Geometry: final body of the model. Coordinates: model frame, mm. Coordinates: 2 decimals unless noted, no trailing zeros. Write item = value, one per line. Start each with the question number.
Autodesk Inventor part; units mm, degrees
ref_plane "YZ Plane" through (0, 0, 0) normal (1, 0, 0) x (0, 1, 0)
ref_plane "XZ Plane" through (0, 0, 0) normal (0, 1, 0) x (-1, 0, 0)
ref_plane "XY Plane" through (0, 0, 0) normal (0, 0, 1) x (1, 0, 0)
sketch "Sketch1" plane through (0, 0, 0) normal (0, 0, 1) x (1, 0, 0)
  line L0 (0, -144.3376) -> (-125, 72.1688) construction
  line L1 (-125, 72.1688) -> (125, 72.1688) construction
  line L2 (125, 72.1688) -> (0, -144.3376) construction
  line L3 (0, 173.2051) -> (150, -86.6025) construction
  line L4 (150, -86.6025) -> (-150, -86.6025) construction
  line L5 (-150, -86.6025) -> (0, 173.2051) construction
  circle A0 centre (-150, -86.6025) radius 1.5875
  circle A1 centre (150, -86.6025) radius 1.5875
  circle A2 centre (0, 173.2051) radius 1.5875
  circle A3 centre (-125, 72.1688) radius 4.25
  circle A4 centre (125, 72.1688) radius 4.25
  circle A5 centre (0, -144.3376) radius 4.25
  circle A6 centre (-150, -86.6025) radius 25 construction
  line L6 (-250.0151, -144.3463) -> (0, 288.6926) construction
  line L7 (0, 288.6926) -> (250.0151, -144.3463) construction
  line L8 (250.0151, -144.3463) -> (-250.0151, -144.3463) construction
  arc A7 (-225.5835, -102.5089) -> (-201.5671, -144.1066) centre (-197.7721, -114.1838) ccw
  circle A8 centre (-125, 72.1688) radius 12.5 construction
  arc A9 (24.0164, 246.6155) -> (-24.0164, 246.6155) centre (0, 228.3676) ccw
  arc A10 (201.5671, -144.1066) -> (225.5835, -102.5089) centre (197.7721, -114.1838) ccw
  arc A11 (-24.0164, 246.6155) -> (-225.5835, -102.5089) centre (1251.5935, -722.6079) ccw
  arc A12 (225.5835, -102.5089) -> (24.0164, 246.6155) centre (-1251.5935, -722.6079) ccw
  arc A13 (-201.5671, -144.1066) -> (201.5671, -144.1066) centre (0, 1445.2157) ccw
  circle A14 centre (0, 228.3676) radius 1.5875
  circle A15 centre (-197.7721, -114.1838) radius 1.5875
  circle A16 centre (197.7721, -114.1838) radius 1.5875
  point P0 (0, 0)
  point P1 (0, 0)
  point P2 (0, 0)
  point P3 (0, 0)
  dimension "d0" = 300
  dimension "d1" = 250
  dimension "d2" = 3.175
  dimension "d3" = 8.5
  dimension "d4" = 50
  dimension "d5" = 60.325
  dimension "d6" = 25
  dimension "d9" = 3.175
extrude "Extrusion2" add sketch "Sketch1" along normal blind 12.5 contours A3 | A4 | A5 | A11 A9 A12 A10 A13 A7
sketch "Sketch8" plane through (0, 0, 12.5) normal (0, 0, 1) x (1, 0, 0)
  circle A0 centre (0, 173.2051) radius 1.5875
  line L0 (15.5, 157.7051) -> (-15.5, 157.7051) construction
  line L1 (-15.5, 157.7051) -> (-15.5, 188.7051) construction
  line L2 (-15.5, 188.7051) -> (15.5, 188.7051) construction
  line L3 (15.5, 188.7051) -> (15.5, 157.7051) construction
  circle A1 centre (-15.5, 157.7051) radius 1.6
  circle A2 centre (15.5, 188.7051) radius 1.6
  point P0 (0, 0)
  dimension "d34" = 3.2
  dimension "d36" = 31
extrude "Extrusion9" cut sketch "Sketch8" against normal through all contours A1 | A2
pattern_circular "Circular Pattern1" count 3 over 360 about axis through (0, 0, -10) along (0, 0, 1) of "Extrusion9"
sketch "Sketch9" plane through (0, 0, 0) normal (0, 0, -1) x (-1, 0, 0)
  circle A0 centre (43.0398, -61.7471) radius 1.621
  circle A1 centre (11.3411, 93.1567) radius 1.621
  circle A2 centre (-31.9602, 68.1567) radius 1.621
  circle A3 centre (86.3411, -36.7471) radius 1.621
  line L0 (-76.356, 80.0525) -> (31.144, -106.143)
  line L1 (31.144, -106.143) -> (130.7369, -48.643)
  line L2 (130.7369, -48.643) -> (23.2369, 137.5525)
  line L3 (23.2369, 137.5525) -> (-76.356, 80.0525)
  line L4 (-51.5025, -76.895) -> (-72.9929, -89.3025)
  arc A4 (-79.8231, -87.4724) -> (-72.9929, -89.3025) centre (-75.4929, -84.9724) ccw
  line L5 (-79.8231, -87.4724) -> (-115.6621, -25.3974)
  arc A5 (-113.8319, -18.5673) -> (-115.6621, -25.3974) centre (-111.3319, -22.8974) ccw
  line L6 (-113.8319, -18.5673) -> (-92.3415, -6.1598)
  arc A6 (-85.5114, -7.9899) -> (-92.3415, -6.1598) centre (-89.8415, -10.4899) ccw
  line L7 (-85.5114, -7.9899) -> (-49.6724, -70.0649)
  arc A7 (-51.5025, -76.895) -> (-49.6724, -70.0649) centre (-54.0025, -72.5649) ccw
  circle A8 centre (-41.0253, -76.0422) radius 1.5
  circle A9 centre (-78.9702, -97.9497) radius 1.5
  circle A10 centre (-86.3643, 2.4873) radius 1.5
  arc A11 (-125.8092, -16.8221) -> (-126.9072, -20.9202) centre (-124.3092, -19.4202) ccw
  line L8 (-126.9072, -20.9202) -> (-81.5682, -99.4497)
  arc A12 (-81.5682, -99.4497) -> (-77.4702, -100.5477) centre (-78.9702, -97.9497) ccw
  line L9 (-77.4702, -100.5477) -> (-39.5253, -78.6402)
  arc A13 (-39.5253, -78.6402) -> (-38.4272, -74.5422) centre (-41.0253, -76.0422) ccw
  line L10 (-38.4272, -74.5422) -> (-83.7662, 3.9873)
  arc A14 (-83.7662, 3.9873) -> (-87.8643, 5.0854) centre (-86.3643, 2.4873) ccw
  line L11 (-87.8643, 5.0854) -> (-125.8092, -16.8221)
  circle A15 centre (-124.3092, -19.4202) radius 1.5
  point P0 (0, 0)
extrude "Extrusion10" cut sketch "Sketch9" against normal through all contours A0 | A1 | A2 | A3 | A8 | A9 | A10 | A15
fillet "Fillet2" radius 6.35 6 edges at (0, 258.5301, 0) (135.8253, 78.4188, 0) (223.8936, -129.265, 0) (0, -156.8376, 0) (-223.8936, -129.265, 0) (-135.8253, 78.4188, 0)
sketch "Sketch2" plane through (0, 0, 12.5) normal (0, 0, 1) x (1, 0, 0)
  circle A0 centre (0, 0) radius 105
  dimension "d12" = 210
sketch "Sketch3" plane through (0, 0, 10.595) normal (0, 0, 1) x (1, 0, 0)
  circle A0 centre (0, 0) radius 105
  line L0 (-31.25, 100.2419) -> (-31.25, 30)
  line L1 (-31.25, 30) -> (31.25, 30)
  line L2 (31.25, 30) -> (31.25, 100.2419)
  line L3 (0, 30) -> (0, 105) construction
  dimension "d16" = 75
  dimension "d18" = 62.5
sketch "Sketch4" plane through (0, 0, 12.5) normal (0, 0, 1) x (1, 0, 0)
  circle A0 centre (0, 0) radius 105
  circle A1 centre (0, 105) radius 12.5
  dimension "d21" = 25
sketch "Sketch5" plane through (0, 0, 12.5) normal (0, 0, 1) x (1, 0, 0)
  arc A0 (24.0164, 246.6155) -> (-24.0164, 246.6155) centre (0, 228.3676) ccw
  arc A1 (201.5671, -144.1066) -> (225.5835, -102.5089) centre (197.7721, -114.1838) ccw
  circle A2 centre (0, 228.3676) radius 1.5875
  circle A3 centre (-197.7721, -114.1838) radius 1.5875
  circle A4 centre (197.7721, -114.1838) radius 1.5875
  circle A5 centre (0, 228.3676) radius 30.1625
  circle A6 centre (197.7721, -114.1838) radius 30.1625
  circle A7 centre (-197.7721, -114.1838) radius 30.1625
sketch "Sketch6" plane through (-193.442, -111.6838, 571.3) normal (0, 0, 1) x (1, 0, 0)
  circle A0 centre (0, 0) radius 1.5875
  circle A1 centre (0, 0) radius 30.1625
  arc A2 (205.9198, 215.9397) -> (180.9642, 215.9397) centre (193.442, 216.6838) ccw
  arc A3 (180.9642, 215.9397) -> (205.9198, 215.9397) centre (193.442, 111.6838) ccw
  circle A4 centre (193.442, -32.6538) radius 4.25
  circle A5 centre (318.442, 183.8526) radius 4.25
  circle A6 centre (68.442, 183.8526) radius 4.25
  circle A7 centre (193.442, 284.8889) radius 1.5875
  circle A8 centre (343.442, 25.0812) radius 1.5875
  circle A9 centre (43.442, 25.0812) radius 1.5875
  arc A10 (-4.6471, -29.8024) -> (-28.1332, 10.8766) centre (0, 0) ccw
  arc A11 (-4.6471, -29.8024) -> (391.5311, -29.8024) centre (193.442, 1240.5571) ccw
  arc A12 (415.0172, 10.8766) -> (391.5311, -29.8024) centre (386.884, 0) ccw
  arc A13 (415.0172, 10.8766) -> (216.928, 353.9771) centre (-784.1909, -452.7528) ccw
  arc A14 (169.956, 353.9771) -> (216.928, 353.9771) centre (193.442, 335.0514) ccw
  arc A15 (169.956, 353.9771) -> (-28.1332, 10.8766) centre (1171.0749, -452.7528) ccw
  circle A16 centre (193.442, 335.0514) radius 1.5875
  circle A17 centre (193.442, 335.0514) radius 30.1625
  circle A18 centre (386.884, 0) radius 1.5875
  circle A19 centre (386.884, 0) radius 30.1625
sketch "Sketch7" plane through (-193.442, -111.6838, -89.1) normal (0, 0, -1) x (-1, 0, 0)
  circle A0 centre (0, 0) radius 30.1625
  circle A1 centre (-68.442, 183.8526) radius 4.25
  circle A2 centre (-318.442, 183.8526) radius 4.25
  circle A3 centre (-193.442, -32.6538) radius 4.25
  circle A4 centre (-43.442, 25.0812) radius 1.5875
  circle A5 centre (-343.442, 25.0812) radius 1.5875
  circle A6 centre (-193.442, 284.8889) radius 1.5875
  circle A7 centre (-386.884, 0) radius 1.5875
  circle A8 centre (-193.442, 335.0514) radius 1.5875
  circle A9 centre (0, 0) radius 1.5875
  arc A10 (-169.956, 353.9771) -> (-216.928, 353.9771) centre (-193.442, 335.0514) ccw
  arc A11 (28.1332, 10.8766) -> (-169.956, 353.9771) centre (-1171.0749, -452.7528) ccw
  arc A12 (-391.5311, -29.8024) -> (4.6471, -29.8024) centre (-193.442, 1240.5571) ccw
  arc A13 (-415.0172, 10.8766) -> (-391.5311, -29.8024) centre (-386.884, 0) ccw
  arc A14 (-216.928, 353.9771) -> (-415.0172, 10.8766) centre (784.1909, -452.7528) ccw
  arc A15 (4.6471, -29.8024) -> (28.1332, 10.8766) centre (0, 0) ccw
  point P0 (-193.442, 111.6838)
properties part number "BOT PLATE"
Item 1: Line query: line 1 (Y direction, x = 150, z = 6.25) (3 decimals); line 2 (X direction, y = 228, z = 7); line 3 (Z direction, x = 107, y = 115). Output: solid intervals per line, ascending. Write a range as from..to.
Item 2: Section query A-A (z = 2.5). Count the separate pieces of the cut face and the enclosed holes in it, plus the area to 3 significant figures.
Item 3: First-contact query: pin 1 (3.5 mm diameter, centred on x = 41.03, y = -76.04, fed in from -Z); pin 2 (2.5 mm diameter, centred on x = 0, y = 173.21, fed in from -Z); pin 3 (4 mm diameter, centred on y = -21, z = 10.5, fed in from -X). Flat tips, straight axial feed; report the tip coordinate or a pass-through.
Verdict:
q1.line_1 = -149.799..-88.19, -85.015..53.348
q1.line_2 = -37.95..-1.54, 1.54..37.95
q1.line_3 = 0.01..12.5
q2.separate_pieces = 1
q2.enclosed_holes = 20
q2.area = 114,000 mm2
q3.pin_1 = 0
q3.pin_2 = through
q3.pin_3 = -189.63
